CAD build for the part. Positions are in the model's coordinates, mm. Face numbers are marked on the shaded views. A direction names the side the tool comes from. Coordinates: 2 decimals unless noted, no trailing zeros. Loops run counter-clockwise (first coordinate to the right, second up) from the corner with the lowest first, then second, coordinate; pieces in that order, holes last.
1) Saw through at B-B, the plane y = 10. Write the cut outline in (x, z).
2) Two-plate mould, pull along X, no slides. Class the marked faces 1, 2 and 3: +X half, -X half, draft (parallel to the pull), parting line (faces both ways), or undercut.
3) Saw through at A-A, the plane z = 0. Write the cut outline in (x, y), and give its area (3 significant figures).
4) Saw through at C-C, the plane z = 4.5. Write the cut outline in (x, y), and give its area (3 significant figures).
5) Saw through at D-D, the plane x = -6. Write the cut outline in (y, z) (3 decimals), and give its area (3 significant figures).
6) Wall check: line 1 along Y through (x, z) = (-1.25, 0); line 2 along X through (y, z) = (1.8, 6); line 3 along Z through (x, y) = (3.25, 10). Give the ranges that are in metal, low to high.
7) Pin check, flat tip, straight feed: pin 1 Ø0.7 at (x, z) = (5, 7) entering from -Y. Stop position of the tip, or through.
8) Which spindle directions (+Z, -Z, +X, -X, +Y, -Y) get a long thin tool onto all of the face, cutting with end or side? Do the marked faces 4 and 5. Say none if no direction does.
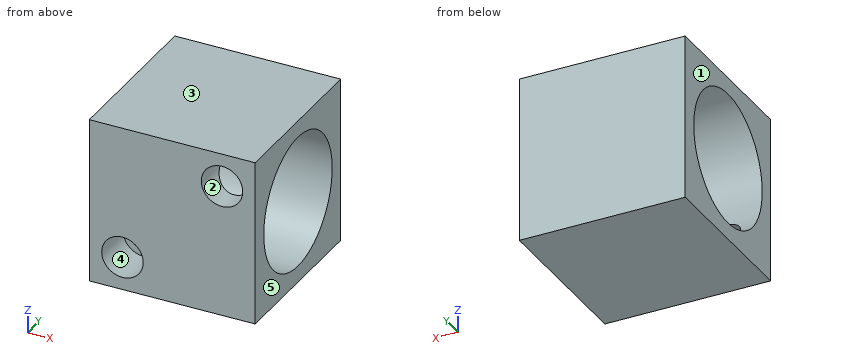
```python
from build123d import *

# Parameters (mm, degrees)
SKETCH1_W               = 20
SKETCH1_H               = 20
BOSS_EXTRUDE1_DEPTH     = 20
SKETCH2_R               = 8
CUT_EXTRUDE1_DEPTH      = 20
CUT_EXTRUDE1_DEPTH_BACK = 20
SKETCH3_R               = 2.5
CUT_EXTRUDE2_DEPTH      = 5


with BuildPart() as part:
    # Sketch1 → Boss-Extrude1 (new body)
    with BuildSketch(Plane(origin=(0, 0, 0), x_dir=(1, 0, 0), z_dir=(0, 1, 0))):
        Rectangle(SKETCH1_W, SKETCH1_H)
    extrude(amount=BOSS_EXTRUDE1_DEPTH)

    # Sketch2 → Cut-Extrude1 (cut, two sides)
    with BuildSketch(Plane(origin=(0, 0, 0), x_dir=(0, 0, -1), z_dir=(1, 0, 0))) as cut_extrude1_sk:
        with Locations((0, 10)):
            Circle(SKETCH2_R)
    extrude(amount=CUT_EXTRUDE1_DEPTH, mode=Mode.SUBTRACT)
    extrude(cut_extrude1_sk.sketch, amount=-CUT_EXTRUDE1_DEPTH_BACK, mode=Mode.SUBTRACT)

    # Sketch3 → Cut-Extrude2 (cut)
    with BuildSketch(Plane(origin=(0, 0, 0), x_dir=(-1, 0, 0), z_dir=(0, -1, 0))):
        with Locations((-6, -6)):
            Circle(SKETCH3_R)
        with Locations((6, 6)):
            Circle(SKETCH3_R)
    extrude(amount=-CUT_EXTRUDE2_DEPTH, mode=Mode.SUBTRACT)


solid = part.part
```
Data:
1. outline: (-10, -10) - (10, -10) - (10, -8) - (-10, -8) - close; (-10, 8) - (10, 8) - (10, 10) - (-10, 10) - close
2. face 1: -X half
2. face 2: undercut
2. face 3: draft
3. outline: (-10, 0) - (10, 0) - (10, 2) - (-10, 2) - close; (-10, 18) - (10, 18) - (10, 20) - (-10, 20) - close
3. area: 80.0 mm2
4. outline: (-10, 0) - (4, 0) - (4, 3.39) - (-10, 3.39) - close; (-10, 16.61) - (10, 16.61) - (10, 20) - (-10, 20) - close; (8, 0) - (10, 0) - (10, 3.39) - (8, 3.39) - close
4. area: 122 mm2
5. outline: (0, -10) - (20, -10) - (20, 10) - (0, 10) - (0, -3.5) - (2.806, -3.5) arc R8 cw (long way) to (5, -6.245) - (5, -8.5) - (0, -8.5) - close
5. area: 177 mm2
6. line 1: y = 0 to 2, 18 to 20
6. line 2: x = -10 to 3.5, 8.5 to 10
6. line 3: z = -10 to -8, 8 to 10
7. pin 1: stops at y = 5
8. face 4: -Y
8. face 5: +Z, -Z, +X, +Y, -Y
